Check sheet for the modelled part. Datum: model origin and axes. Units: mm. Face numbers are marked on the shaded views. Give positions to 0.01 mm unless a question says otherwise; leave off trailing zeros. Write each loop counter-clockwise with the first axis right and the second up, starting at its lowest first coordinate (ties: lowest second). Pieces come first, ordered by that corner, then holes. Notation, with made-up numbers: (-21.5, -40) -> (23.5, -40) arc R8 cw to (23.5, -31) -> close; hole circle Ø9 at (-11, 39.25). An arc over 180 degrees is marked (long way). Use a Markdown table: item, result. Add a question column.
1. Scan lines: probe 1 along Z at (x, y) = (1.25, 1); probe 2 along X at (y, z) = (1.2, -0.15); probe 3 along X at (y, z) = (0.85, -5.5). Record each from-to range of solid material in increasing order. Write a range as [from, to].
2. Cross-section at C-C (y = 0.85). Enter the section's corners in (x, z).
3. Release check for a two-part mould opening along X. For the marked faces 1, 2 and 3 record: released by +X, released by -X, zero draft, split by the parting line, or undercut.
4. Cross-section at D-D (x = 5.5). Enter the section's corners in (y, z), then the cut area to 3 significant figures.
5. Cross-section at A-A (z = -2.69). Enter the section's corners in (x, y).
6. Cross-section at B-B (x = 0). Enter the section's corners in (y, z), then the cut area to 3 significant figures.
7. Gauge pin test, flat ends, axial feed: P1, Ø1.8, axis at x = 0, z = 4.5, coming from the -Y side; P2, Ø3, axis at x = 2, z = 4.5, coming from the -Y side. Record the tip position at first contact, or that the pin passes through.
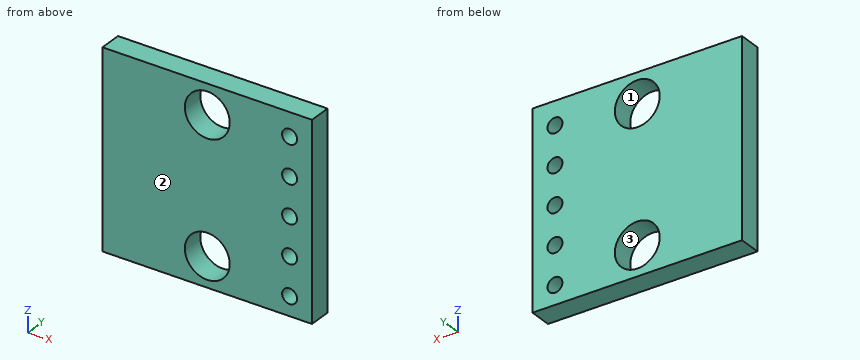
from build123d import *

# Parameters (mm, degrees)
SKETCH1_W           = 14
SKETCH1_H           = 13
BOSS_EXTRUDE1_DEPTH = 1.5
SKETCH2_R           = 1.5
SKETCH2_R_2         = 0.5
CUT_EXTRUDE1_DEPTH  = 1.5


with BuildPart() as part:
    # Sketch1 → Boss-Extrude1 (new body)
    with BuildSketch(Plane(origin=(0, 0, 0), x_dir=(1, 0, 0), z_dir=(0, 1, 0))):
        Rectangle(SKETCH1_W, SKETCH1_H)
    extrude(amount=BOSS_EXTRUDE1_DEPTH)

    # Sketch2 → Cut-Extrude1 (cut)
    with BuildSketch(Plane(origin=(0, 1.5, 0), x_dir=(1, 0, 0), z_dir=(0, 1, 0))):
        with Locations(Location((0, 4.5, 0), (0, 0, 270))):
            Circle(SKETCH2_R)
        with Locations(Location((0, -4.5, 0), (0, 0, 270))):
            Circle(SKETCH2_R)
        with Locations(Location((5.5, -4.93, 0), (0, 0, 270))):
            Circle(SKETCH2_R_2)
        with Locations(Location((5.5, -2.39, 0), (0, 0, 270))):
            Circle(SKETCH2_R_2)
        with Locations(Location((5.5, 0.15, 0), (0, 0, 270))):
            Circle(SKETCH2_R_2)
        with Locations(Location((5.5, 2.69, 0), (0, 0, 270))):
            Circle(SKETCH2_R_2)
        with Locations(Location((5.5, 5.23, 0), (0, 0, 270))):
            Circle(SKETCH2_R_2)
    extrude(amount=-CUT_EXTRUDE1_DEPTH, mode=Mode.SUBTRACT)


solid = part.part
Worked answers:
| question | item | result |
|---|---|---|
| 1 | probe 1 | z = [-6.5, -5.33], [-3.67, 3.67], [5.33, 6.5] |
| 1 | probe 2 | x = [-7, 5], [6, 7] |
| 1 | probe 3 | x = [-7, -1.12], [1.12, 5.08], [5.92, 7] |
| 2 | outline | (-7, -6.5) -> (7, -6.5) -> (7, 6.5) -> (-7, 6.5) -> close; hole circle Ø3 at (0, -4.5); hole circle Ø3 at (0, 4.5); hole circle Ø1 at (5.5, -5.23); hole circle Ø1 at (5.5, -2.69); hole circle Ø1 at (5.5, -0.15); hole circle Ø1 at (5.5, 2.39); hole circle Ø1 at (5.5, 4.93) |
| 3 | face 1 | undercut |
| 3 | face 2 | zero draft |
| 3 | face 3 | undercut |
| 4 | outline | (0, -6.5) -> (1.5, -6.5) -> (1.5, -5.73) -> (0, -5.73) -> close; (0, -4.73) -> (1.5, -4.73) -> (1.5, -3.19) -> (0, -3.19) -> close; (0, -2.19) -> (1.5, -2.19) -> (1.5, -0.65) -> (0, -0.65) -> close; (0, 0.35) -> (1.5, 0.35) -> (1.5, 1.89) -> (0, 1.89) -> close; (0, 2.89) -> (1.5, 2.89) -> (1.5, 4.43) -> (0, 4.43) -> close; (0, 5.43) -> (1.5, 5.43) -> (1.5, 6.5) -> (0, 6.5) -> close |
| 4 | area | 12.0 mm² |
| 5 | outline | (-7, 0) -> (5, 0) -> (5, 1.5) -> (-7, 1.5) -> close; (6, 0) -> (7, 0) -> (7, 1.5) -> (6, 1.5) -> close |
| 6 | outline | (0, -6.5) -> (1.5, -6.5) -> (1.5, -6) -> (0, -6) -> close; (0, -3) -> (1.5, -3) -> (1.5, 3) -> (0, 3) -> close; (0, 6) -> (1.5, 6) -> (1.5, 6.5) -> (0, 6.5) -> close |
| 6 | area | 10.5 mm² |
| 7 | P1 | passes through |
| 7 | P2 | stops at y = 0 |
